Verification items for the finished model (mm, model axes). Face numbers are marked on the shaded views. A direction names the side the tool comes from. Coordinates: 2 decimals unless noted, no trailing zeros. Write each loop counter-clockwise with the first axis right and the second up, starting at its lowest first coordinate (ties: lowest second). Pieces come first, ordered by that corner, then holes. Notation, with made-up numbers: (31, 15.5) -> (64, 15.5) arc R14 ccw to (64, 28.5) -> close; hole circle Ø8 at (4.5, 33.5). An arc over 180 degrees is marked (long way). Use a Markdown table: item, result. Add a question column.
from build123d import *

# Parameters (mm, degrees)
SKETCH1_W           = 100
SKETCH1_H           = 100
BOSS_EXTRUDE1_DEPTH = 7.5
FILLET1_R           = 15
SKETCH2_R           = 5.625
CUT_EXTRUDE1_DEPTH  = 7.5
SKETCH3_R           = 27.5
BOSS_EXTRUDE2_DEPTH = 2.5
SKETCH5_W           = 40
SKETCH5_H           = 10
BOSS_EXTRUDE4_DEPTH = 40
SKETCH6_R           = 5
CUT_EXTRUDE2_DEPTH  = 10
CUT_EXTRUDE3_DEPTH  = 1.875


with BuildPart() as part:
    # Sketch1 → Boss-Extrude1 (new body)
    with BuildSketch(Plane(origin=(0, 0, 0), x_dir=(1, 0, 0), z_dir=(0, 1, 0))):
        Rectangle(SKETCH1_W, SKETCH1_H)
    extrude(amount=BOSS_EXTRUDE1_DEPTH)

    # Fillet1
    fillet1_edges = [part.edges().sort_by_distance(p)[0] for p in [
        (50, 3.75, 50),
        (-50, 3.75, 50),
        (-50, 3.75, -50),
        (50, 3.75, -50),
    ]]
    fillet(fillet1_edges, radius=FILLET1_R)

    # Sketch2 → Cut-Extrude1 (cut)
    with BuildSketch(Plane(origin=(0, 7.5, 0), x_dir=(1, 0, 0), z_dir=(0, 1, 0))):
        with Locations(Location((-35, 35, 0), (0, 0, 270))):
            Circle(SKETCH2_R)
        with Locations(Location((35, 35, 0), (0, 0, 90))):
            Circle(SKETCH2_R)
        with Locations(Location((35, -35, 0), (0, 0, 270))):
            Circle(SKETCH2_R)
        with Locations(Location((-35, -35, 0), (0, 0, 90))):
            Circle(SKETCH2_R)
    extrude(amount=-CUT_EXTRUDE1_DEPTH, mode=Mode.SUBTRACT)

    # Sketch3 → Boss-Extrude2 (add)
    with BuildSketch(Plane(origin=(0, 7.5, 0), x_dir=(1, 0, 0), z_dir=(0, 1, 0))):
        with Locations(Location((0, 0, 0), (0, 0, 270))):
            Circle(SKETCH3_R)
    extrude(amount=BOSS_EXTRUDE2_DEPTH)

    # Sketch5 → Boss-Extrude4 (add)
    with BuildSketch(Plane(origin=(0, 10, 0), x_dir=(1, 0, 0), z_dir=(0, 1, 0))):
        with Locations((0, -11.25)):
            Rectangle(SKETCH5_W, SKETCH5_H)
    boss_extrude4 = extrude(amount=BOSS_EXTRUDE4_DEPTH)

    # Sketch6 → Cut-Extrude2 (cut)
    with BuildSketch(Plane.XY.offset(16.25)):
        with BuildLine():
            ThreePointArc((10.462689665, 34.134564665), (0, 41.25), (-10.462689665, 34.134564665))
            Line((-10.462689665, 34.134564665), (-20, 10))
            Line((-20, 10), (-20, 50))
            Line((-20, 50), (20, 50))
            Line((20, 50), (20, 10))
            Line((20, 10), (10.462689665, 34.134564665))
        make_face()
        with Locations((0, 30)):
            Circle(SKETCH6_R)
    cut_extrude2 = extrude(amount=-CUT_EXTRUDE2_DEPTH, mode=Mode.SUBTRACT)

    # Mirror4: Boss-Extrude4, Cut-Extrude2 across plane
    add(boss_extrude4.mirror(Plane.XY))
    add(cut_extrude2.mirror(Plane.XY), mode=Mode.SUBTRACT)

    # Sketch7 → Cut-Extrude3 (cut)
    with BuildSketch(Plane.XZ):
        with BuildLine():
            Line((-20, -25), (20, -25))
            ThreePointArc((20, -25), (23.535533906, -23.535533906), (25, -20))
            Line((25, -20), (25, 20))
            ThreePointArc((25, 20), (23.535533906, 23.535533906), (20, 25))
            Line((20, 25), (-20, 25))
            ThreePointArc((-20, 25), (-23.535533906, 23.535533906), (-25, 20))
            Line((-25, 20), (-25, -20))
            ThreePointArc((-25, -20), (-23.535533906, -23.535533906), (-20, -25))
        make_face()
    extrude(amount=-CUT_EXTRUDE3_DEPTH, mode=Mode.SUBTRACT)


solid = part.part
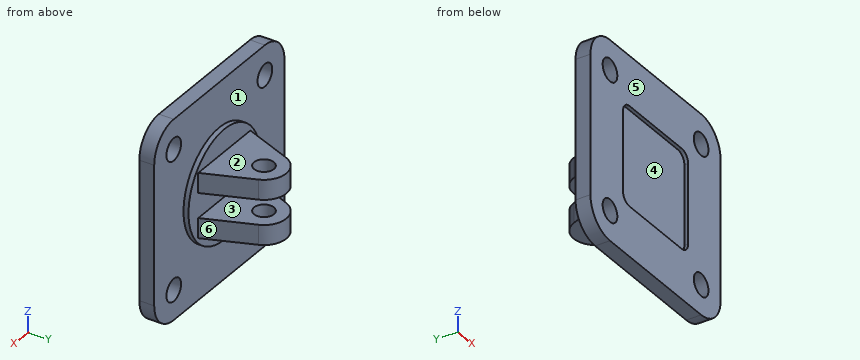
1) Cross-section at B-B on y = 5. Record the boundary of the cut face in (x, z) (3 decimals).
2) Cross-section at D-D on z = 0. Record the boundary of the cut face in (x, y) (3 decimals).
3) Thickness scan on L1, parallel to X at y = 4.75, z = -35 (3 decimals); L2, parallel to Z at x = 5, y = 18.5; L3, parallel to Y at x = 0, z = -11.25 (3 decimals). Record the ranges inside material, lowest first.
4) Release check for a two-part mould opening along X. For the marked faces 4, 5 and 6 record: released by +X, released by -X, zero draft, split by the parting line, or undercut.
5) Cross-section at C-C on y = 11.5. Record the boundary of the cut face in (x, z), then the cut area to 3 significant figures.
6) Set-up check for the marked faces 1, 2 and 3: record each of +Z, -Z, +X, -X, +Y, -Y from which the full face is reachable in a straight line by a thin tool's end or side.
7) Gauge pin test, flat ends, axial feed: pin 1 (4 mm diameter, centred on x = 11.5, y = 23.5, fed in from -Z); pin 2 (15 mm diameter, centred on x = -0.5, z = -5, fed in from -Y) (3 decimals); pin 3 (6 mm diameter, centred on x = -37.5, z = -13.5, fed in from +Y). Record the tip position at first contact, or that the pin passes through.
8) Cross-section at A-A on x = 0. Record the boundary of the cut face in (y, z) (3 decimals).
Returned:
| question | item | result |
|---|---|---|
| 1 | outline | (-50, -35) arc R15 ccw to (-35, -50) -> (35, -50) arc R15 ccw to (50, -35) -> (50, 35) arc R15 ccw to (35, 50) -> (-35, 50) arc R15 ccw to (-50, 35) -> close; hole circle Ø11.25 at (-35, -35); hole circle Ø11.25 at (-35, 35); hole circle Ø11.25 at (35, -35); hole circle Ø11.25 at (35, 35) |
| 2 | outline | (-50, 0) -> (-25, 0) -> (-25, 1.875) -> (25, 1.875) -> (25, 0) -> (50, 0) -> (50, 7.5) -> (27.5, 7.5) -> (27.5, 10) -> (-27.5, 10) -> (-27.5, 7.5) -> (-50, 7.5) -> close |
| 3 | L1 | x = -50 to -40.625, -29.375 to 29.375, 40.625 to 50 |
| 3 | L2 | z = -16.25 to -6.25, 6.25 to 16.25 |
| 3 | L3 | y = 1.875 to 25, 35 to 41.25 |
| 4 | face 4 | undercut |
| 4 | face 5 | zero draft |
| 4 | face 6 | released by +X |
| 5 | outline | (-19.41, -16.25) -> (19.41, -16.25) -> (19.41, -6.25) -> (-19.41, -6.25) -> close; (-19.41, 6.25) -> (19.41, 6.25) -> (19.41, 16.25) -> (-19.41, 16.25) -> close |
| 5 | area | 776 mm² |
| 6 | face 1 | +Y |
| 6 | face 2 | +Z, +X, -X, +Y |
| 6 | face 3 | +X, -X, +Y |
| 7 | pin 1 | stops at z = -16.25 |
| 7 | pin 2 | stops at y = 1.875 |
| 7 | pin 3 | stops at y = 7.5 |
| 8 | outline | (0, -50) -> (7.5, -50) -> (7.5, -27.5) -> (10, -27.5) -> (10, -16.25) -> (25, -16.25) -> (25, -6.25) -> (10, -6.25) -> (10, 6.25) -> (25, 6.25) -> (25, 16.25) -> (10, 16.25) -> (10, 27.5) -> (7.5, 27.5) -> (7.5, 50) -> (0, 50) -> (0, 25) -> (1.875, 25) -> (1.875, -25) -> (0, -25) -> close; (35, -16.25) -> (41.25, -16.25) -> (41.25, -6.25) -> (35, -6.25) -> close; (35, 6.25) -> (41.25, 6.25) -> (41.25, 16.25) -> (35, 16.25) -> close |
